from build123d import *

# Parameters (mm, degrees)
F0_R     = 11.049
F1_DEPTH = 2.54
F2_R     = 5.461
F3_DEPTH = 3.81
F4_R     = 3.9878
F4_R_2   = 2.334094
F5_DEPTH = 6.35


with BuildPart() as f1:
    # F0 (on Top) → F1 (new body)
    with BuildSketch(Plane.XY):
        Circle(F0_R)
    extrude(amount=F1_DEPTH)

    # F2 (on Top) → F3 (join)
    with BuildSketch(Plane.XY):
        Circle(F2_R)
    extrude(amount=F3_DEPTH)

    # F4 (on Top) → F5 (join)
    with BuildSketch(Plane.XY):
        Circle(F4_R)
        Circle(F4_R_2, mode=Mode.SUBTRACT)
    extrude(amount=F5_DEPTH)


solid = f1.part
Input: part model. Units: mm. Frame: model coordinates. A direction names the side the tool comes from. Give positions to 0.01 mm unless a question says otherwise; leave off trailing zeros. Loops run counter-clockwise (first coordinate to the right, second up) from the corner with the lowest first, then second, coordinate; pieces in that order, holes last. Notation, with made-up numbers: (72, 35) -> (104, 35) arc R35 cw to (104, 72) -> close; hole circle Ø6 at (-12.5, -11.5). An arc over 180 degrees is marked (long way). Answer as a JSON object with one key per item and string values. Group by question number.
Item 1: Line query: probe 1 along Y at (x, z) = (0, 4.6); probe 2 along Z at (x, y) = (5.75, -0.5). Output: solid intervals per line, ascending.
Item 2: Cut plane C-C, the plane z = 5. Return the cut outline in (x, y), and give its area (3 significant figures).
Item 3: Cut plane D-D, the plane z = 2.25. Return the cut outline in (x, y).
Item 4: Reachability of faces 5 (the flat face through (-4, -2, 3.81)), 6 (the flat face through (0, 0, 0)) from +Z, -Z, +X, -X, +Y, -Y: full face, straight path, thin tool, end or side. Return the list, or none.
Item 5: Cut plane A-A, the plane x = 0. Return the cut outline in (y, z), and give its area (3 significant figures).
Item 6: Pin query (flat end, axial travel): P1, Ø1, axis at x = -8.5, y = -5, coming from the -Z side; P2, Ø1.4, axis at x = 0.5, y = 1, coming from the +Z side; P3, Ø2, axis at y = 1, z = 4.5, coming from the -X side. Return the tip coordinate at first contact, or that it passes through.
Item 7: Pull-direction query (X, two-part tool) for faces 1 (the flat face through (2, -2, 6.35)), 2 (the cylindrical face through (-2.33, 0.1, 5.06)), 3 (the cylindrical face through (-1.438, 10.955, 1.252)), 4 (the flat face through (0, 0, 3.81)); classes: released by +X, released by -X, zero draft, split by the parting line, or undercut.
Checks:
{
 "1": {"probe 1": "y = -3.99 to -2.33, 2.33 to 3.99", "probe 2": "z = 0 to 2.54"},
 "2": {"outline": "circle Ø7.98 at (0, 0); hole circle Ø4.67 at (0, 0)", "area": "32.8 mm²"},
 "3": {"outline": "circle Ø22.1 at (0, 0)"},
 "4": {"face 5": "+Z", "face 6": "-Z, +X, -X, +Y, -Y"},
 "5": {"outline": "(-11.05, 0) -> (11.05, 0) -> (11.05, 2.54) -> (5.46, 2.54) -> (5.46, 3.81) -> (3.99, 3.81) -> (3.99, 6.35) -> (2.33, 6.35) -> (2.33, 3.81) -> (-2.33, 3.81) -> (-2.33, 6.35) -> (-3.99, 6.35) -> (-3.99, 3.81) -> (-5.46, 3.81) -> (-5.46, 2.54) -> (-11.05, 2.54) -> close", "area": "78.4 mm²"},
 "6": {"P1": "stops at z = 0", "P2": "stops at z = 3.81", "P3": "stops at x = -5.45"},
 "7": {"face 1": "zero draft", "face 2": "undercut", "face 3": "split by the parting line", "face 4": "undercut"}
}
